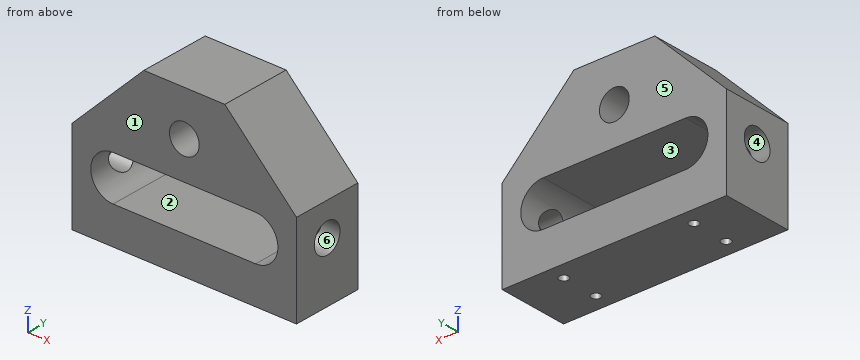
from build123d import *

# Parameters (mm, degrees)
SKETCH_R          = 4
PAD_DEPTH         = 9.525
SKETCH001_R       = 4
POCKET_DEPTH      = 30.152111
POCKET_DEPTH_BACK = 30.152111
SKETCH003_R       = 1.25
HOLE_DEPTH        = 8
HOLE_TIPS_R       = 1.25


with BuildPart() as part:
    # Sketch → Pad (new body, symmetric)
    with BuildSketch(Plane.XZ):
        Polygon((-10.880411, 28.06969), (10.880411, 28.06969), (30.151111, 8.79899), (30.151111, -16), (-30.151111, -16), (-30.151111, 8.79899), align=None)
        with Locations((0, 16.06969)):
            Circle(SKETCH_R, mode=Mode.SUBTRACT)
        with BuildLine():
            ThreePointArc((-19.151111, 6), (-25.151111, 0), (-19.151111, -6))
            Line((-19.151111, -6), (19.151111, -6))
            ThreePointArc((19.151111, -6), (25.151111, 0), (19.151111, 6))
            Line((19.151111, 6), (-19.151111, 6))
        make_face(mode=Mode.SUBTRACT)
    extrude(amount=PAD_DEPTH, both=True)

    # Sketch001 → Pocket (cut, two sides)
    with BuildSketch(Plane.YZ) as pocket_sk:
        Circle(SKETCH001_R)
    extrude(amount=-POCKET_DEPTH, mode=Mode.SUBTRACT)
    extrude(pocket_sk.sketch, amount=POCKET_DEPTH_BACK, mode=Mode.SUBTRACT)

    # Sketch003 → Hole (cut)
    with BuildSketch(Plane.XY.offset(-16)):
        with Locations((-17.5, 5)):
            Circle(SKETCH003_R)
        with Locations((-17.5, -5)):
            Circle(SKETCH003_R)
        with Locations((17.5, -5)):
            Circle(SKETCH003_R)
        with Locations((17.5, 5)):
            Circle(SKETCH003_R)
    extrude(amount=HOLE_DEPTH, mode=Mode.SUBTRACT)

    # Hole tips → Hole tip 1 section 0
    with BuildSketch(Plane.XY.offset(-8), mode=Mode.PRIVATE) as hole_tip_1_s0:
        with Locations((-17.5, 5)):
            Circle(HOLE_TIPS_R)
    loft([hole_tip_1_s0.sketch, Vertex(-17.5, 5, -7.248924)], mode=Mode.SUBTRACT)

    # Hole tips → Hole tip 2 section 0
    with BuildSketch(Plane.XY.offset(-8), mode=Mode.PRIVATE) as hole_tip_2_s0:
        with Locations((-17.5, -5)):
            Circle(HOLE_TIPS_R)
    loft([hole_tip_2_s0.sketch, Vertex(-17.5, -5, -7.248924)], mode=Mode.SUBTRACT)

    # Hole tips → Hole tip 3 section 0
    with BuildSketch(Plane.XY.offset(-8), mode=Mode.PRIVATE) as hole_tip_3_s0:
        with Locations((17.5, -5)):
            Circle(HOLE_TIPS_R)
    loft([hole_tip_3_s0.sketch, Vertex(17.5, -5, -7.248924)], mode=Mode.SUBTRACT)

    # Hole tips → Hole tip 4 section 0
    with BuildSketch(Plane.XY.offset(-8), mode=Mode.PRIVATE) as hole_tip_4_s0:
        with Locations((17.5, 5)):
            Circle(HOLE_TIPS_R)
    loft([hole_tip_4_s0.sketch, Vertex(17.5, 5, -7.248924)], mode=Mode.SUBTRACT)


solid = part.part
Input: part model. Units: mm. Frame: model coordinates. Face numbers are marked on the shaded views. A direction names the side the tool comes from. Give positions to 0.01 mm unless a question says otherwise; leave off trailing zeros. Order: outer loops, then holes, each group sorted by start corner. A loop starts at its lowest first (then second) coordinate and runs counter-clockwise, first axis right, second up. Notation, with made-up numbers: M 74,80 L 88,80 A21 cw 88,119 Z; hole C 25,-36.5 d7. An arc over 180 degrees is marked long. Answer as a JSON object with one key per item and string values.
1. First-contact query: P1, Ø4, axis at x = 17.5, y = 5, coming from the +Z side; P2, Ø6, axis at y = -2.5, z = 12, coming from the +X side; P3, Ø2, axis at x = 17.5, y = -5, coming from the -Z side. Flat tips, straight axial feed; report the tip coordinate or a pass-through.
Result sheet:
{"P1": "z = 23.45", "P2": "x = 29.95", "P3": "z = -7.85"}
2. Cut plane C-C, the plane x = 7. Output: boundary loops of the cut face in (y, z) (3 decimals).
Result sheet:
{"outline": "M -9.525,-16 L 9.525,-16 L 9.525,-6 L -9.525,-6 Z; M -9.525,6 L 9.525,6 L 9.525,28.07 L -9.525,28.07 Z"}
3. Cut plane A-A, the plane z = 0. Output: boundary loops of the cut face in (x, y) (3 decimals), and give its area (4 significant figures).
Result sheet:
{"outline": "M -30.151,-9.525 L -25.151,-9.525 L -25.151,-4 L -30.151,-4 Z; M -30.151,4 L -25.151,4 L -25.151,9.525 L -30.151,9.525 Z; M 25.151,-9.525 L 30.151,-9.525 L 30.151,-4 L 25.151,-4 Z; M 25.151,4 L 30.151,4 L 30.151,9.525 L 25.151,9.525 Z", "area": "110.5 mm²"}
4. Pull-direction query (Y, two-part tool) for the marked faces 3, 4, 5 and 6; classes: +Y half, -Y half, draft (parallel to the pull), parting line (faces both ways), or undercut.
Result sheet:
{"face 3": "draft", "face 4": "undercut", "face 5": "+Y half", "face 6": "undercut"}
5. Cut plane D-D, the plane y = 0.25. Output: boundary loops of the cut face in (x, z), and give its area (3 significant figures).
Result sheet:
{"outline": "M -30.15,-16 L 30.15,-16 L 30.15,-3.99 L 23.63,-3.99 A6 cw 19.15,-6 L -19.15,-6 A6 cw -23.63,-3.99 L -30.15,-3.99 Z; M -30.15,3.99 L -23.63,3.99 A6 cw -19.15,6 L 19.15,6 A6 cw 23.63,3.99 L 30.15,3.99 L 30.15,8.8 L 10.88,28.07 L -10.88,28.07 L -30.15,8.8 Z; hole C 0,16.07 d8", "area": "1,580 mm²"}
6. Cut plane B-B, the plane x = 0. Output: boundary loops of the cut face in (y, z) (3 decimals), and give its area (3 significant figures).
Result sheet:
{"outline": "M -9.525,-16 L 9.525,-16 L 9.525,-6 L -9.525,-6 Z; M -9.525,6 L 9.525,6 L 9.525,12.07 L -9.525,12.07 Z; M -9.525,20.07 L 9.525,20.07 L 9.525,28.07 L -9.525,28.07 Z", "area": "459 mm²"}
7. Ray query, line 1 (Z direction, x = 0, y = 1.75); line 2 (Y direction, x = -27.25, z = 0) (3 decimals); line 3 (Z direction, x = -10.5, y = -7.5). Return the intervals inside material, ascending. Write a range as [from, to].
Result sheet:
{"line 1": "[-16, -6], [6, 12.07], [20.07, 28.07]", "line 2": "[-9.525, -4], [4, 9.525]", "line 3": "[-16, -6], [6, 28.07]"}
8. Reachability of the marked faces 1 and 2 from +Z, -Z, +X, -X, +Y, -Y: full face, straight path, thin tool, end or side. Return the list, or none.
Result sheet:
{"face 1": "+Z, -Z, +X, -X, -Y", "face 2": "+Y, -Y"}
